Source: three-view drawing plus pictorial views. Frame: mm from the lowest corner of the part. Coordinates: 2 decimals unless noted, no trailing zeros. Write each loop counter-clockwise with the first axis right and the second up, starting at its lowest first coordinate (ties: lowest second). Pieces come first, ordered by that corner, then holes. Notation, with made-up numbers: (50, 31) - (79, 31) arc R25 ccw to (79, 64) - close; hole circle Ø1 at (42, 4.25). An arc over 180 degrees is marked (long way). Put each result on its own line as item: value.
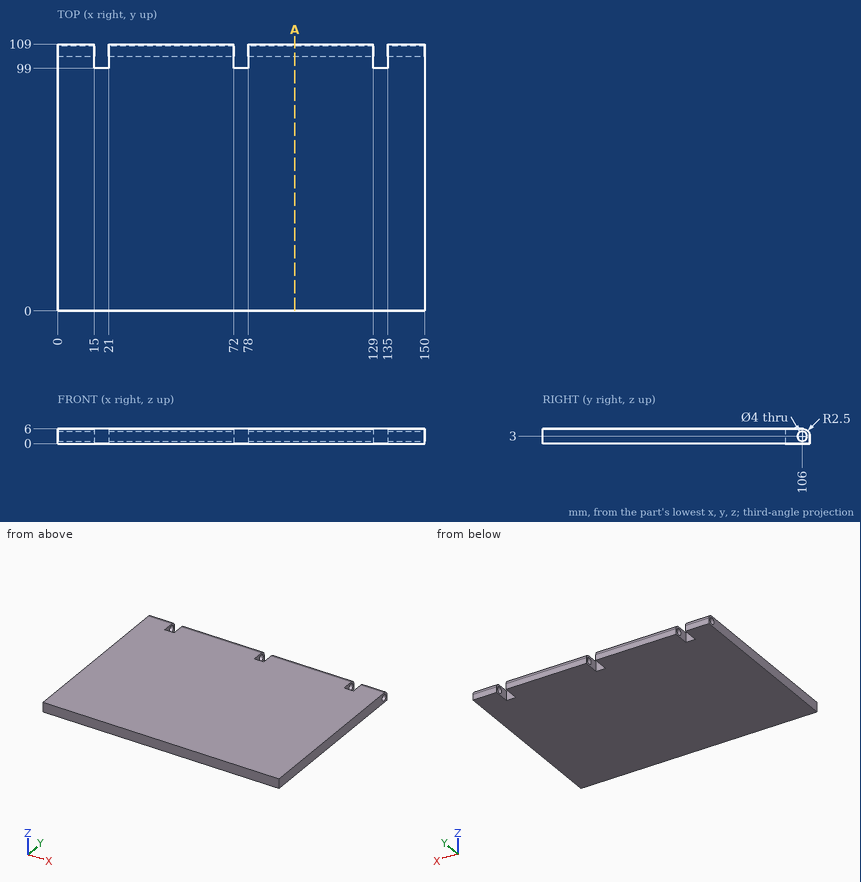
1. Pin query (flat end, axial travel): pin 1 Ø3 at (y, z) = (106, 2) entering from +X; pin 2 Ø3 at (x, z) = (131.5, 4) entering from +Y. Return the tip coordinate at first contact, or that it passes through.
Answer below:
pin 1: stops at x = 150
pin 2: stops at y = 99
2. Section query A-A (x = 97). Return loops of the section in (y, z), then the cut area to 3 significant figures.
Answer below:
outline: (0, 0) - (109, 0) - (109, 3.5) arc R2.5 ccw to (106.5, 6) - (0, 6) - close; hole circle Ø4 at (106, 3)
area: 640 mm²
3. Ray query, probe 1 along X at (y, z) = (101, 4.1); probe 2 along Z at (x, y) = (94, 106); probe 3 along Y at (x, z) = (44, 2.4). Return the intervals inside material, ascending. Write a range as from..to.
Answer below:
probe 1: x = 0..15, 21..72, 78..129, 135..150
probe 2: z = 0..1, 5..6
probe 3: y = 0..104.09, 107.91..109
